from build123d import *

# Parameters (mm, degrees)
SKETCH2_W           = 30
SKETCH2_H           = 35
BOSS_EXTRUDE1_DEPTH = 2
FILLET1_R           = 5
SKETCH3_R           = 2
CUT_EXTRUDE1_DEPTH  = 10
SKETCH6_R           = 4
BOSS_EXTRUDE2_DEPTH = 30
FILLET2_R           = 1


with BuildPart() as part:
    # Sketch2 → Boss-Extrude1 (new body)
    with BuildSketch(Plane.XY):
        with Locations((15, -17.5)):
            Rectangle(SKETCH2_W, SKETCH2_H)
    extrude(amount=BOSS_EXTRUDE1_DEPTH)

    # Fillet1
    fillet1_edges = [part.edges().sort_by_distance(p)[0] for p in [
        (0, 0, 1),
        (30, 0, 1),
        (30, -35, 1),
        (0, -35, 1),
    ]]
    fillet(fillet1_edges, radius=FILLET1_R)

    # Sketch3 → Cut-Extrude1 (cut)
    with BuildSketch(Plane.XY.offset(2)):
        with Locations((6, -5.5)):
            Circle(SKETCH3_R)
        with Locations((24, -5.5)):
            Circle(SKETCH3_R)
        with Locations((6, -29.5)):
            Circle(SKETCH3_R)
        with Locations((24, -29.5)):
            Circle(SKETCH3_R)
    extrude(amount=-CUT_EXTRUDE1_DEPTH, mode=Mode.SUBTRACT)

    # Sketch6 → Boss-Extrude2 (add)
    with BuildSketch(Plane(origin=(0, 0, 0), x_dir=(-1, 0, 0), z_dir=(0, 0, -1))):
        with Locations((-15, -17.5)):
            Circle(SKETCH6_R)
    extrude(amount=BOSS_EXTRUDE2_DEPTH)

    # Fillet2
    fillet2_edges = [part.edges().sort_by_distance(p)[0] for p in [
        (19, -17.5, -30),
    ]]
    fillet(fillet2_edges, radius=FILLET2_R)


solid = part.part
The listing builds one solid part. Answer for the finished solid, in the listing's coordinates (mm). Round coordinates to 2 decimals unless told otherwise and drop trailing zeros. Order: outer loops, then holes, each group sorted by start corner. A loop starts at its lowest first (then second) coordinate and runs counter-clockwise, first axis right, second up. Notation, with made-up numbers: (31.25, 15) - (57.25, 15) arc R30 cw to (57.25, 50) - close; hole circle Ø3 at (6.5, 30). An arc over 180 degrees is marked (long way). Write item = value, one per line. Start each with the question number.
1) For a pull along X with two mould halves and no side action, classify faces 1 (the cylindrical face through (4.4, -6.7, 1)), 2 (the cylindrical face through (17.95, -14.8, -14.3)), 3 (the flat face through (15, 0, 1)), 4 (the cylindrical face through (1, -2, 1)) as released by +X, released by -X, zero draft, split by the parting line, or undercut.
2) Straight lines are drawn through the part: L1, parallel to Y at x = 24, z = 1.5; L2, parallel to Z at x = 4.5, y = -23; L3, parallel to X at y = -29, z = 1. For each, find the intervals that lie inside material, in ascending order.
3) Given pin 1 (4.5 mm diameter, centred on x = 6, y = -29.5, fed in from -Z); pin 2 (5 mm diameter, centred on x = 4, z = -3, fed in from +Y); pin 3 (12 mm diameter, centred on y = -17, z = -10, fed in from -X); pin 4 (8 mm diameter, centred on y = -22.5, z = -18.5, fed in from -X), each flat-ended and moving along its own axis, determine where each tip first touches the part or whether it passes through.
4) Section D-D, the plane z = -5.5 is taken. Write down the section's boundary in (x, y), plus the area to 3 significant figures.
5) Section C-C, the plane y = -17.5 is taken. Write down the section's boundary in (x, z), plus the area to 3 significant figures.
6) Section B-B, the plane x = 6 is taken. Write down the section's boundary in (y, z).
7) Section A-A, the plane y = -29.5 is taken. Write down the section's boundary in (x, z), plus the area to 3 significant figures.
Results list:
q1.face_1 = undercut
q1.face_2 = split by the parting line
q1.face_3 = zero draft
q1.face_4 = released by -X
q2.L1 = -35 to -31.5, -27.5 to -7.5, -3.5 to 0
q2.L2 = 0 to 2
q2.L3 = 0 to 4.06, 7.94 to 22.06, 25.94 to 30
q3.pin_1 = 0
q3.pin_2 = through
q3.pin_3 = 11
q3.pin_4 = 11.13
q4.outline = circle Ø8 at (15, -17.5)
q4.area = 50.3 mm^2
q5.outline = (0, 0) - (11, 0) - (11, -29) arc R1 ccw to (12, -30) - (18, -30) arc R1 ccw to (19, -29) - (19, 0) - (30, 0) - (30, 2) - (0, 2) - close
q5.area = 300 mm^2
q6.outline = (-35, 0) - (-31.5, 0) - (-31.5, 2) - (-35, 2) - close; (-27.5, 0) - (-7.5, 0) - (-7.5, 2) - (-27.5, 2) - close; (-3.5, 0) - (0, 0) - (0, 2) - (-3.5, 2) - close
q7.outline = (0, 0) - (4, 0) - (4, 2) - (0, 2) - close; (8, 0) - (22, 0) - (22, 2) - (8, 2) - close; (26, 0) - (30, 0) - (30, 2) - (26, 2) - close
q7.area = 44.0 mm^2
